Could you check a few things on this model? Use its own coordinates, in mm. A direction names the side the tool comes from. Give positions to 0.01 mm unless a question says otherwise; leave off trailing zeros. Loops run counter-clockwise (first coordinate to the right, second up) from the corner with the lowest first, then second, coordinate; pieces in that order, holes last. Notation, with made-up numbers: M 28,-25 L 68,-25 A16 ccw 68,-21 Z; hole C -6.5,-11.5 d10. An arc over 180 degrees is marked long. Use CSV: the item, a comma, the result in double quotes.
```python
from build123d import *

# Parameters (mm, degrees)
SKETCH002_W   = 44.6
SKETCH002_H   = 24.4
SKETCH002_W_2 = 40.6
SKETCH002_H_2 = 20.4
PAD001_DEPTH  = 12
PAD003_DEPTH  = 2
PAD_DEPTH     = 5
SKETCH005_W   = 9
SKETCH005_H   = 22
SKETCH005_W_2 = 5
SKETCH005_H_2 = 17
PAD004_DEPTH  = 5
SKETCH012_W   = 44.6
SKETCH012_H   = 24.4
SKETCH012_W_2 = 36
SKETCH012_H_2 = 18.4
PAD011_DEPTH  = 10


with BuildPart() as part:
    # Sketch002 → Pad001 (new body)
    with BuildSketch(Plane.XY):
        with Locations((20.3, 10.2)):
            Rectangle(SKETCH002_W, SKETCH002_H)
        with Locations((20.3, 10.2)):
            Rectangle(SKETCH002_W_2, SKETCH002_H_2, mode=Mode.SUBTRACT)
    extrude(amount=PAD001_DEPTH)

    # Sketch004 → Pad003 (join)
    with BuildSketch(Plane.XZ):
        Polygon((0, 12), (17.8, -12.5), (22.8, -12.5), (40.6, 12), align=None)
    extrude(amount=PAD003_DEPTH)

    # Sketch → Pad (join)
    with BuildSketch(Plane(origin=(17.8, 0, 10), x_dir=(0, 1, 0), z_dir=(1, 0, 0))):
        with BuildLine():
            Line((-22, 12), (-22, 0))
            ThreePointArc((-22, 0), (-20.991352, -2.812026), (-19.211103, -5.211103))
            Line((-19.211103, -5.211103), (-2, -22.422205))
            Line((-2, -22.422205), (-2, 2))
            Line((-2, 12), (-2, 2))
            Line((-5, 12), (-2, 12))
            Line((-5, 2), (-5, 12))
            ThreePointArc((-19, 2), (-12, -5), (-5, 2))
            Line((-19, 12), (-19, 2))
            Line((-22, 12), (-19, 12))
        make_face()
    extrude(amount=PAD_DEPTH)

    # Sketch005 → Pad004 (join)
    with BuildSketch(Plane(origin=(17.8, 0, 22), x_dir=(1, 0, 0), z_dir=(0, 0, 1))):
        with Locations((2.5, -11)):
            Rectangle(SKETCH005_W, SKETCH005_H)
        with Locations((2.5, -10.5)):
            Rectangle(SKETCH005_W_2, SKETCH005_H_2, mode=Mode.SUBTRACT)
    extrude(amount=-PAD004_DEPTH)

    # Sketch012 → Pad011 (join)
    with BuildSketch(Plane.XY.offset(12)):
        with Locations((20.3, 10.2)):
            Rectangle(SKETCH012_W, SKETCH012_H)
        with Locations((20, 11.2)):
            Rectangle(SKETCH012_W_2, SKETCH012_H_2, mode=Mode.SUBTRACT)
    extrude(amount=PAD011_DEPTH)


solid = part.part
```
1. Please list where these lines run through material, in increasing order: line 1 (Y direction, x = 9, z = 13); line 2 (X direction, y = -13, z = 17.5); line 3 (Y direction, x = 13, z = 8.5).
Outcome:
line 1,"-2 to 2, 20.4 to 22.4"
line 2,"15.8 to 17.8, 22.8 to 24.8"
line 3,"-2 to 0, 20.4 to 22.4"
2. If we mould it in two halves opening along X, with no side actions, what happens to faces 4 (the face through (17.8, -12, 20)), 5 (the face through (27.277, -0.986, -6.337)), 6 (the face through (20, 22.4, 11))? For each: +X half, -X half, draft (parallel to the pull), parting line (faces both ways), or undercut.
Outcome:
face 4,"undercut"
face 5,"+X half"
face 6,"draft"
3. I want a section at C-C, the plane y = -12. List the corners of the cut face in (x, z) for me.
Outcome:
outline,"M 15.8,17 L 17.8,17 L 17.8,22 L 15.8,22 Z; M 17.8,-2.42 L 22.8,-2.42 L 22.8,5 L 17.8,5 Z; M 22.8,17 L 24.8,17 L 24.8,22 L 22.8,22 Z"
4. I'm going to push flat-ended pins straight in: pin 1 Ø10.5 at (x, z) = (13.5, 2.5) entering from -Y; pin 2 Ø12.5 at (x, z) = (18, -3.5) entering from +Y; pin 3 Ø1 at (x, y) = (23.5, -17) entering from -Z; pin 4 Ø1.5 at (y, z) = (-14, 18.5) entering from +X. Where does each tip first touch, or does it pass through?
Outcome:
pin 1,"y = -19.87"
pin 2,"y = 22.4"
pin 3,"z = 17"
pin 4,"x = 24.8"
5. I want a section at D-D, the plane x = 24. List the corners of the cut face in (y, z) for me, then the cut area to 3 significant figures.
Outcome:
outline,"M -22,17 L -2,17 L -2,-10.85 L 0,-10.85 L 0,12 L 2,12 L 2,22 L -22,22 Z; M 20.4,0 L 22.4,0 L 22.4,22 L 20.4,22 Z"
area,"230 mm2"
6. Which directions (+Z, -Z, +X, -X, +Y, -Y) give clear straight access to the entire face, cutting with the end or side of a thin tool? Please do faces 1 (the face through (17, -12, 17)), 2 (the face through (20, 0, 2)), 3 (the face through (22.8, -10, 2)).
Outcome:
face 1,"-Z, -X, -Y"
face 2,"-Z"
face 3,"-Z, +X, -Y"
7. I want a section at B-B, the plane z = 9. List the corners of the cut face in (x, y) for me.
Outcome:
outline,"M -2,-2 L 17.8,-2 L 17.8,-5.68 L 22.8,-5.68 L 22.8,-2 L 42.6,-2 L 42.6,22.4 L -2,22.4 Z; M 17.8,-21.75 L 22.8,-21.75 L 22.8,-18.32 L 17.8,-18.32 Z; hole M 0,0 L 40.6,0 L 40.6,20.4 L 0,20.4 Z"
8. I want a section at A-A, the plane x = 36. List the corners of the cut face in (y, z) for me, then the cut area to 3 significant figures.
Outcome:
outline,"M -2,0 L 0,0 L 0,12 L 2,12 L 2,22 L -2,22 Z; M 20.4,0 L 22.4,0 L 22.4,22 L 20.4,22 Z"
area,"108 mm2"
